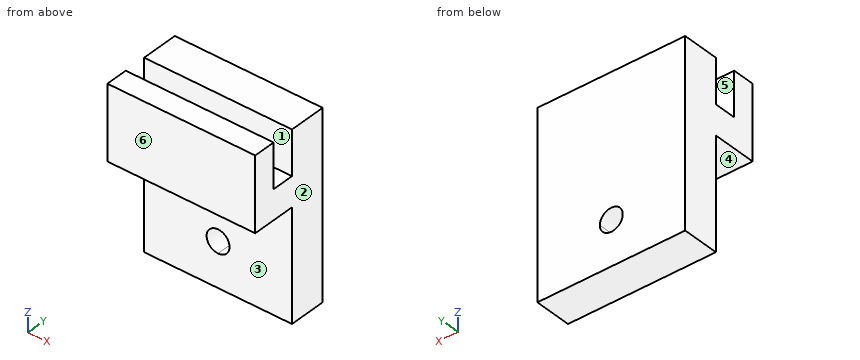
```python
from build123d import *

# Parameters (mm, degrees)
F0_W     = 20
F0_H     = 25
F1_DEPTH = 5
F2_W     = 20
F2_H     = 4
F3_DEPTH = 3
F4_W     = 20
F4_H     = 4
F4_H_2   = 6
F5_DEPTH = 3
F7_DEPTH = 25


with BuildPart() as f1:
    # F0 (on Front) → F1 (new body)
    with BuildSketch(Plane.XZ):
        Rectangle(F0_W, F0_H)
    extrude(amount=F1_DEPTH)

    # F2 (on face) → F3 (join)
    with BuildSketch(Plane.XZ.offset(5)):
        with Locations((0, 4.5)):
            Rectangle(F2_W, F2_H)
    extrude(amount=F3_DEPTH)

    # F4 (on face) → F5 (join)
    with BuildSketch(Plane.XZ.offset(8)):
        with Locations((0, 4.5)):
            Rectangle(F4_W, F4_H)
        with Locations((0, 9.5)):
            Rectangle(F4_W, F4_H_2)
    extrude(amount=F5_DEPTH)

    # F6 (on face) → F7 (cut)
    with BuildSketch(Plane.XZ.offset(5)):
        with BuildLine():
            ThreePointArc((1.55, -6.5), (-1.096016, -5.403984), (0, -8.05))
            ThreePointArc((0, -8.05), (1.096016, -7.596016), (1.55, -6.5))
        make_face()
    extrude(amount=-F7_DEPTH, mode=Mode.SUBTRACT)


solid = f1.part
```
Verification items for the finished model (mm, model axes). Face numbers are marked on the shaded views. A direction names the side the tool comes from. Give positions to 0.01 mm unless a question says otherwise; leave off trailing zeros. Order: outer loops, then holes, each group sorted by start corner. A loop starts at its lowest first (then second) coordinate and runs counter-clockwise, first axis right, second up. Notation, with made-up numbers: M 87.25,87.25 L 119.25,87.25 A22 ccw 119.25,110.25 Z; hole C -21,-27.75 d6. An arc over 180 degrees is marked long. Answer in a Markdown table with one row per item. Add a question column.
Item 1: Section check A-A, the plane x = 8.5. Enter the section's corners in (y, z).
Item 2: Tool access check on the marked faces 4, 5 and 6. Record the directions out of +Z, -Z, +X, -X, +Y, -Y that give a thin tool (end or side, any length) a straight path to the whole face; none if there is none.
Item 3: Section check B-B, the plane y = -4. Enter the section's corners in (x, z), and give its area (3 significant figures).
Item 4: Mould release check, pull along Y, two halves, no side actions. Record for the marked faces 1, 2 and 3: released by +Y, released by -Y, zero draft, split by the parting line, or undercut.
Item 5: Scan lines: probe 1 along Y at (x, z) = (7.75, 8.25); probe 2 along X at (y, z) = (-4, -6.5); probe 3 along Z at (x, y) = (0, -1.15). Record each from-to range of solid material in increasing order. Write a range as from..to.
Item 6: Section check C-C, the plane z = -7.5. Enter the section's corners in (x, y), and give its area (3 significant figures).
Item 7: Section check D-D, the plane x = -1. Enter the section's corners in (y, z).
Item 8: Gauge pin test, flat ends, axial feed: pin 1 (2.5 mm diameter, centred on x = 0.5, y = -6.5, fed in from +Z); pin 2 (5 mm diameter, centred on x = 2, y = -9.5, fed in from -Z). Record the tip position at first contact, or that the pin passes through.
Filled sheet:
| question | item | result |
|---|---|---|
| 1 | outline | M -11,2.5 L -5,2.5 L -5,-12.5 L 0,-12.5 L 0,12.5 L -5,12.5 L -5,6.5 L -8,6.5 L -8,12.5 L -11,12.5 Z |
| 2 | face 4 | -Z, +X, -X, -Y |
| 2 | face 5 | +Z, +X, -X |
| 2 | face 6 | +Z, -Z, +X, -X, -Y |
| 3 | outline | M -10,-12.5 L 10,-12.5 L 10,12.5 L -10,12.5 Z; hole M 0,-8.05 A1.55 ccw 1.55,-6.5 A1.55 ccw long Z |
| 3 | area | 492 mm^2 |
| 4 | face 1 | undercut |
| 4 | face 2 | zero draft |
| 4 | face 3 | released by -Y |
| 5 | probe 1 | y = -11..-8, -5..0 |
| 5 | probe 2 | x = -10..-1.55, 1.55..10 |
| 5 | probe 3 | z = -12.5..-8.05, -4.95..12.5 |
| 6 | outline | M -10,-5 L -1.18,-5 L -1.18,0 L -10,0 Z; M 1.18,-5 L 10,-5 L 10,0 L 1.18,0 Z |
| 6 | area | 88.2 mm^2 |
| 7 | outline | M -11,2.5 L -5,2.5 L -5,-5.32 L 0,-5.32 L 0,12.5 L -5,12.5 L -5,6.5 L -8,6.5 L -8,12.5 L -11,12.5 Z; M -5,-12.5 L 0,-12.5 L 0,-7.68 L -5,-7.68 Z |
| 8 | pin 1 | stops at z = 6.5 |
| 8 | pin 2 | stops at z = 2.5 |
